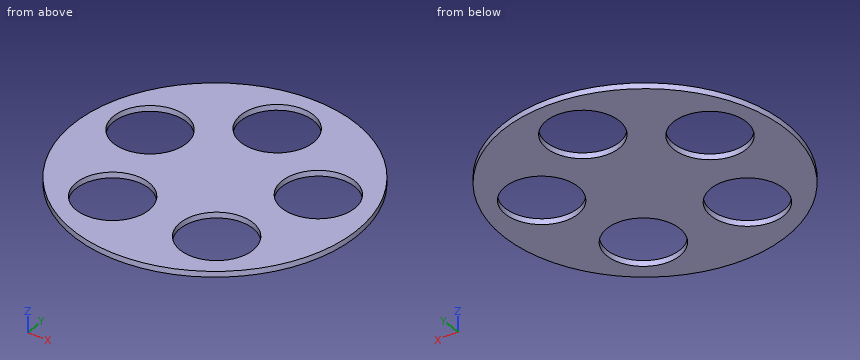
from build123d import *

# Parameters (mm, degrees)
F0_R     = 44.45
F0_R_2   = 11.43
F1_DEPTH = 1.778


with BuildPart() as f1:
    # F0 (on Top) → F1 (new body)
    with BuildSketch(Plane.XY):
        Circle(F0_R)
        with Locations((-16.42272, -22.603935)):
            Circle(F0_R_2, mode=Mode.SUBTRACT)
        with Locations((16.42272, -22.603935)):
            Circle(F0_R_2, mode=Mode.SUBTRACT)
        with Locations((-26.572519, 8.633935)):
            Circle(F0_R_2, mode=Mode.SUBTRACT)
        with Locations((26.572519, 8.633935)):
            Circle(F0_R_2, mode=Mode.SUBTRACT)
        with Locations((0, 27.94)):
            Circle(F0_R_2, mode=Mode.SUBTRACT)
    extrude(amount=F1_DEPTH)


solid = f1.part
Verification items for the finished model (mm, model axes). Coordinates: 2 decimals unless noted, no trailing zeros. Order: outer loops, then holes, each group sorted by start corner. A loop starts at its lowest first (then second) coordinate and runs counter-clockwise, first axis right, second up. Notation, with made-up numbers: (-20.5, 48) -> (-13.5, 48) arc R14 cw to (-13.5, 62) -> close; hole circle Ø1 at (-28.75, -17). An arc over 180 degrees is marked (long way). Put each result on its own line as item: value. Start each with the question number.
1. Cross-section at A-A, the plane x = 0. Record the boundary of the cut face in (y, z).
2. Cross-section at D-D, the plane z = 0.7. Record the boundary of the cut face in (x, y).
3. Material ranges on L1, parallel to X at y = -25, z = 1.2; L2, parallel to Y at x = 19, z = 1.1; L3, parallel to Y at x = -17, z = 1.1, recorded low to high. Write a range as [from, to].
4. Cross-section at B-B, the plane y = 27.94. Record the boundary of the cut face in (x, z), then the cut area to 3 significant figures.
5. Cross-section at C-C, the plane y = 0. Record the boundary of the cut face in (x, z).
Computed:
1. outline: (-44.45, 0) -> (16.51, 0) -> (16.51, 1.78) -> (-44.45, 1.78) -> close; (39.37, 0) -> (44.45, 0) -> (44.45, 1.78) -> (39.37, 1.78) -> close
2. outline: circle Ø88.9 at (0, 0); hole circle Ø22.86 at (-26.57, 8.63); hole circle Ø22.86 at (-16.42, -22.6); hole circle Ø22.86 at (0, 27.94); hole circle Ø22.86 at (16.42, -22.6); hole circle Ø22.86 at (26.57, 8.63)
3. L1: [-36.75, -27.6], [-5.25, 5.25], [27.6, 36.75]
3. L2: [-40.18, -33.74], [-11.47, 0.07], [17.2, 40.18]
3. L3: [-41.07, -34.02], [-11.19, 2.39], [14.88, 41.07]
4. outline: (-34.57, 0) -> (-11.43, 0) -> (-11.43, 1.78) -> (-34.57, 1.78) -> close; (11.43, 0) -> (34.57, 0) -> (34.57, 1.78) -> (11.43, 1.78) -> close
4. area: 82.3 mm2
5. outline: (-44.45, 0) -> (-34.06, 0) -> (-34.06, 1.78) -> (-44.45, 1.78) -> close; (-19.08, 0) -> (19.08, 0) -> (19.08, 1.78) -> (-19.08, 1.78) -> close; (34.06, 0) -> (44.45, 0) -> (44.45, 1.78) -> (34.06, 1.78) -> close
